Read the model definition and answer for the solid it produces. Units are mm, in the model's axes. A direction names the side the tool comes from. Give positions to 0.01 mm unless a question says otherwise; leave off trailing zeros. Loops run counter-clockwise (first coordinate to the right, second up) from the corner with the lowest first, then second, coordinate; pieces in that order, holes last. Notation, with made-up numbers: (51, -21.75) - (99, -21.75) arc R35 ccw to (99, 16.25) - close; hole circle Ø4 at (-25, 58.5). An arc over 180 degrees is marked (long way). Put each result on its own line as item: value. Start each with the question number.
1. Consider L1, parallel to Z at x = 679.5, y = -402.5; L2, parallel to Z at x = -153.5, y = -340; L3, parallel to X at y = -313, z = -31. Determine where each line is inside the solid, lowest interval first. Write a range as from..to.
2. Given pin 1 Ø10 at (x, y) = (-88, -49) entering from +Z; pin 2 Ø6 at (y, z) = (-326.5, -217) entering from -X; pin 3 Ø1.5 at (x, y) = (-163.5, -109.5) entering from -Z, each flat-ended and moving along its own axis, determine where each tip first touches the part or whether it passes through.
3. For faces 5 (the cylindrical face through (911.018, -243.331, -334.335)), 6 (the flat face through (111, 0, -331)), 7 (the flat face through (-96.162, -238.548, 16.663)), determine the directions among +Z, -Z, +X, -X, +Y, -Y from which every point of the face is accessible in a straight line to the end or side of a thin tool.
4. A cutting plane is placed at D-D, the plane x = 486.5. Determine the outline of the cut face in (y, z), plus the area to 3 significant figures.
5. A cutting plane is placed at A-A, the plane x = 663.5. Determine the outline of the cut face in (y, z) (3 decimals).
6. A cutting plane is placed at C-C, the plane x = -122. Determine the outline of the cut face in (y, z), plus the area to 3 significant figures.
7. For a pull along Z with two mould halves and no side action, classify faces 1 (the flat face through (399, -239, -310.543)), 2 (the cylindrical face through (-371.68, -238.55, -305.22)), 3 (the cylindrical face through (-13.78, -405.91, 133.65)), 4 (the flat face through (719, -305.435, -334)) as released by +Z, released by -Z, zero draft, split by the parting line, or undercut.
8. A cutting plane is placed at B-B, the plane y = -288. Determine the outline of the cut face in (x, z).
```python
from build123d import *

# Parameters (mm, degrees)
F1_DEPTH = 483.87
F2_R     = 63.5
F3_DEPTH = 52.173089771
F4_R     = 38.1
F5_DEPTH = 50.8
F6_R     = 127
F7_R     = 127
F8_DEPTH = 52.173089771


with BuildPart() as f1:
    # F0 (on Front) → F1 (new body)
    with BuildSketch(Plane.XZ):
        with BuildLine():
            Line((130.1338967539, 242.9592923321), (96.0089234939, 277.0842655921))
            Line((96.0089234939, 277.0842655921), (-353.0038825596, -171.9285404613))
            ThreePointArc((-353.0038825596, -171.9285404613), (-370.6647202624, -307.0074831479), (-244.6667798626, -358.8027045558))
            Line((-244.6667798626, -358.8027045558), (1025.3332201374, -358.8027045558))
            Line((1025.3332201374, -358.8027045558), (1025.3332201374, -310.5427045558))
            Line((1025.3332201374, -310.5427045558), (-244.6667798626, -310.5427045558))
            ThreePointArc((-244.6667798626, -310.5427045558), (-324.3924314451, -286.3084555707), (-316.2091160387, -203.3837204605))
            Line((-316.2091160387, -203.3837204605), (130.1338967539, 242.9592923321))
        make_face()
    extrude(amount=F1_DEPTH)

    # F2 (on face) → F3 (cut, through all)
    with BuildSketch(Plane.XY.offset(-310.5427045558)):
        with Locations((212.5332201374, -241.935)):
            Circle(F2_R)
    extrude(amount=-F3_DEPTH, mode=Mode.SUBTRACT)

    # F4 (on face) → F5 (cut)
    with BuildSketch(Plane(origin=(-90.5376710491, 0, 90.5376710491), x_dir=(0, -1, 0), z_dir=(-0.7071067812, 0, 0.7071067812))):
        with Locations((114.3, 73.3167240172)):
            Circle(F4_R)
        with Locations((369.57, 73.3167240172)):
            Circle(F4_R)
    extrude(amount=-F5_DEPTH, mode=Mode.SUBTRACT)

    # F6
    f6_edges = [f1.edges().sort_by_distance(p)[0] for p in [
        (113.07141, 0, 260.021779),
        (113.07141, -483.87, 260.021779),
    ]]
    fillet(f6_edges, radius=F6_R)

    # F7
    f7_edges = [f1.edges().sort_by_distance(p)[0] for p in [
        (1025.33322, 0, -334.672705),
        (1025.33322, -483.87, -334.672705),
    ]]
    fillet(f7_edges, radius=F7_R)

    # F2 (on face) → F8 (cut, through all)
    with BuildSketch(Plane.XY.offset(-310.5427045558)):
        with BuildLine():
            Line((847.5332201374, -178.435), (593.5332201374, -178.435))
            ThreePointArc((593.5332201374, -178.435), (548.6332037777, -197.0202501392), (530.0332201374, -241.914165099))
            ThreePointArc((530.0332201374, -241.914165099), (548.6306760802, -286.8228125584), (593.5332201374, -305.435))
            Line((593.5332201374, -305.435), (847.5332201374, -305.435))
            ThreePointArc((847.5332201374, -305.435), (892.4345007428, -286.8362806053), (911.0332201374, -241.935))
            ThreePointArc((911.0332201374, -241.935), (892.4345007428, -197.0337193947), (847.5332201374, -178.435))
        make_face()
    extrude(amount=-F8_DEPTH, mode=Mode.SUBTRACT)


solid = f1.part
```
Return value:
1. L1: z = -358.8..-310.54
1. L2: z = -358.8..-310.54, -40.67..27.58
1. L3: x = -212.08..-143.83
2. pin 1: stops at z = 98.08
2. pin 2: stops at x = -381.37
2. pin 3: stops at z = -358.8
3. face 5: +Z, -Z
3. face 6: +Z, -Z, +X, -X, +Y
3. face 7: +X, +Y, -Y
4. outline: (-483.87, -358.8) - (0, -358.8) - (0, -310.54) - (-483.87, -310.54) - close
4. area: 23,400 mm2
5. outline: (-483.87, -358.803) - (-305.435, -358.803) - (-305.435, -310.543) - (-483.87, -310.543) - close; (-178.435, -358.803) - (0, -358.803) - (0, -310.543) - (-178.435, -310.543) - close
6. outline: (-483.87, -358.8) - (0, -358.8) - (0, -310.54) - (-483.87, -310.54) - close; (-483.87, -9.17) - (0, -9.17) - (0, 59.08) - (-483.87, 59.08) - close
6. area: 56,400 mm2
7. face 1: undercut
7. face 2: split by the parting line
7. face 3: undercut
7. face 4: zero draft
8. outline: (-353, -171.93) arc R111.76 ccw to (-244.67, -358.8) - (168.83, -358.8) - (168.83, -310.54) - (-244.67, -310.54) arc R65.69 cw to (-316.21, -203.38) - (130.13, 242.96) - (96.01, 277.08) - close; (256.24, -358.8) - (549.84, -358.8) - (549.84, -310.54) - (256.24, -310.54) - close; (891.24, -358.8) - (1025.33, -358.8) - (1025.33, -310.54) - (891.24, -310.54) - close
